Part model, mm, in its own coordinate system. Face numbers are marked on the shaded views. A direction names the side the tool comes from. Coordinates: 2 decimals unless noted, no trailing zeros. Write each loop counter-clockwise with the first axis right and the second up, starting at its lowest first coordinate (ties: lowest second). Pieces come first, ordered by that corner, then holes. Notation, with made-up numbers: (61.5, -29) - (93.5, -29) arc R14 ccw to (93.5, -12) - close; hole circle Ø7 at (31, -18.5). An arc over 180 degrees is marked (long way). Use a Markdown table: item, result.
```python
from build123d import *

# Parameters (mm, degrees)
F1_DEPTH = 25.4


with BuildPart() as f1:
    # F0 (on Front) → F1 (new body)
    with BuildSketch(Plane.XZ):
        Polygon((0, -6.874368), (15.085418, -29.025108), (9.547733, 0), (29.407017, 14.130645), (5.34673, 10.311551), (0, 27.87938), align=None)
    extrude(amount=F1_DEPTH)

    # F2: F1 across plane


with BuildPart() as f1_1:
    add(f1.part)
    add(f1.part.mirror(Plane.YZ))


solid = f1_1.part
```
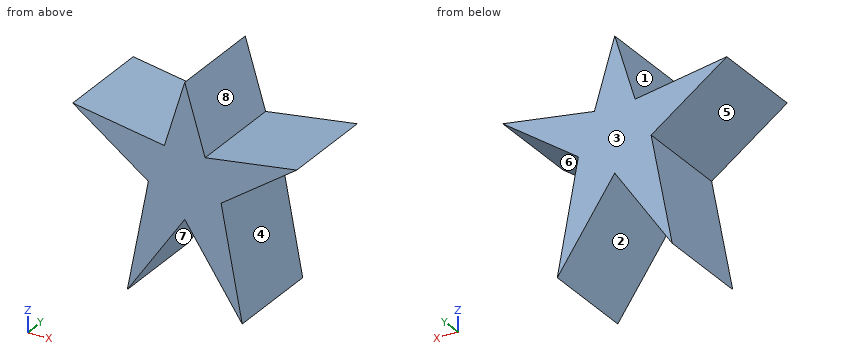
Item 1: Drop flat-ended pins along their axis: P1, Ø5, axis at x = 11.5, y = -7.5, coming from the -Z side; P2, Ø8, axis at x = -20.5, z = 19, coming from the -Y side; P3, Ø8, axis at x = 14.5, y = -20, coming from the +Z side; P4, Ø1, axis at x = -3.5, y = -5, coming from the -Z side. Give the stop position or say it passes through.
From the geometry:
| item | result |
|---|---|
| P1 | z = -27.43 |
| P2 | through |
| P3 | z = 12.4 |
| P4 | z = -12.75 |
Item 2: Which spindle directions (+Z, -Z, +X, -X, +Y, -Y) get a long thin tool onto all of the face, cutting with end or side? Do the marked faces 5, 6, 7 and 8. Say none if no direction does.
From the geometry:
| item | result |
|---|---|
| face 5 | -X, +Y, -Y |
| face 6 | +X, +Y, -Y |
| face 7 | -Z, +Y, -Y |
| face 8 | +Z, +Y, -Y |
Item 3: Band-saw the part on A-A, the plane z = -14. Give the cut face in (x, y).
From the geometry:
| item | result |
|---|---|
| outline | (-12.22, -25.4) - (-4.85, -25.4) - (-4.85, 0) - (-12.22, 0) - close; (4.85, -25.4) - (12.22, -25.4) - (12.22, 0) - (4.85, 0) - close |
Item 4: Band-saw the part on B-B, the plane x = -10.5. Give the cut face in (y, z), then the cut area to 3 significant figures.
From the geometry:
| item | result |
|---|---|
| outline | (-25.4, -22.29) - (0, -22.29) - (0, -4.99) - (-25.4, -4.99) - close; (-25.4, 0.68) - (0, 0.68) - (0, 11.13) - (-25.4, 11.13) - close |
| area | 705 mm^2 |
Item 5: Band-saw the part on C-C, the plane y = -6.25. Give the cut face in (x, z), then the cut area to 3 significant figures.
From the geometry:
| item | result |
|---|---|
| outline | (-29.41, 14.13) - (-9.55, 0) - (-15.09, -29.03) - (0, -6.87) - (15.09, -29.03) - (9.55, 0) - (29.41, 14.13) - (5.35, 10.31) - (0, 27.88) - (-5.35, 10.31) - close |
| area | 892 mm^2 |
Item 6: Drill centre lines: probe 1 along X at (y, z) = (-10.5, -19); probe 2 along X at (y, z) = (-5.75, -7.5); probe 3 along Z at (x, y) = (22.5, -4.25). Where is each one in solid material? Low to high.
From the geometry:
| item | result |
|---|---|
| probe 1 | -13.17 to -8.26, 8.26 to 13.17 |
| probe 2 | -10.98 to -0.43, 0.43 to 10.98 |
| probe 3 | 9.22 to 13.03 |
Item 7: Band-saw the part on D-D, the plane x = 2.5. Give the cut face in (y, z), then the cut area to 3 significant figures.
From the geometry:
| item | result |
|---|---|
| outline | (-25.4, -10.55) - (0, -10.55) - (0, 19.67) - (-25.4, 19.67) - close |
| area | 767 mm^2 |
Item 8: Two-plate mould, pull along X, no slides. Class the marked faces 1, 2, 3 and 4: pulls with the +X half, pulls with the -X half, needs draft (parallel to the pull), parting line crosses it, or undercut.
From the geometry:
| item | result |
|---|---|
| face 1 | undercut |
| face 2 | undercut |
| face 3 | needs draft |
| face 4 | pulls with the +X half |
